Geometry: final body of the model. Coordinates: model frame, mm. A direction names the side the tool comes from. Coordinates: 2 decimals unless noted, no trailing zeros. Order: outer loops, then holes, each group sorted by start corner. A loop starts at its lowest first (then second) coordinate and runs counter-clockwise, first axis right, second up. Notation, with made-up numbers: (18, -5) - (34, -5) arc R31 cw to (34, 25) - close; hole circle Ø1 at (-28.75, 28.25). An arc over 180 degrees is marked (long way). Use a Markdown table: item, result. Add a question column.
```python
from build123d import *

# Parameters (mm, degrees)
F0_W     = 49
F0_H     = 49
F0_W_2   = 41
F0_H_2   = 41
F1_DEPTH = 20
F2_DEPTH = 10
F3_D     = 5.5
F5_D     = 5.5
F7_DEPTH = 5


with BuildPart() as f1:
    # F0 (on Front) → F1 (new body)
    with BuildSketch(Plane.XZ):
        Rectangle(F0_W, F0_H)
        Rectangle(F0_W_2, F0_H_2, mode=Mode.SUBTRACT)
    extrude(amount=F1_DEPTH)

    # F0 (on Front) → F2 (join)
    with BuildSketch(Plane.XZ):
        Rectangle(F0_W, F0_H)
        Rectangle(F0_W_2, F0_H_2, mode=Mode.SUBTRACT)
        Rectangle(F0_W_2, F0_H_2)
    extrude(amount=-F2_DEPTH)

    # F3 (through all)
    with Locations(Plane.XZ):
        with Locations((0, 10), (0, -10)):
            Hole(F3_D / 2)

    # F5 (through all)
    with Locations(Plane.YZ.offset(24.5)):
        with Locations((-10, 0)):
            Hole(F5_D / 2)


with BuildPart() as f7:
    # F6 (on face) → F7 (new body)
    with BuildSketch(Plane.XZ):
        Polygon((5.1, 10), (2.55, 14.4167295593), (-2.55, 14.4167295593), (-5.1, 10), (-2.55, 5.5832704407), (2.55, 5.5832704407), align=None)
    extrude(amount=-F7_DEPTH)


with BuildPart() as f7b:
    # F6 (on face) → F7, piece 2 (new body)
    with BuildSketch(Plane.XZ):
        Polygon((5.1, -10), (2.55, -5.5832704407), (-2.55, -5.5832704407), (-5.1, -10), (-2.55, -14.4167295593), (2.55, -14.4167295593), align=None)
    extrude(amount=-F7_DEPTH)


with BuildPart() as f1_1:
    add(f1.part)

    # F8: cut F7, F7b
    add(f7.part, mode=Mode.SUBTRACT)
    add(f7b.part, mode=Mode.SUBTRACT)


solid = f1_1.part
```
1) Line query: line 1 (Z direction, x = 0, y = 8.05); line 2 (Z direction, x = -15, y = -10.5). Output: solid intervals per line, ascending. Write a range as from..to.
2) Access query for faces 4 (the flat face through (0, -10, 20.5)), 5 (the flat face through (21, -20, 0)). Directions: +Z, -Z, +X, -X, +Y, -Y. A direction counts if a zero-diameter tool reaches every point of the face in a straight line with its end or side. Return the directions, or none.
3) Section query A-A (x = 0). Return the cut outline in (y, z).
4) Section query B-B (y = -10). Return the cut outline in (x, z).
5) Section query D-D (x = -14). Return the cut outline in (y, z).
6) First-contact query: pin 1 (7 mm diameter, centred on x = 0, z = 10, fed in from -Y); pin 2 (8 mm diameter, centred on x = -13, z = -16, fed in from -Y); pin 3 (2.5 mm diameter, centred on x = 1, z = 10.5, fed in from -Y). Flat tips, straight axial feed; report the tip coordinate or a pass-through.
7) Section query C-C (z = 0). Return the cut outline in (x, y), and give its area (3 significant figures).
8) Draft query along Y for faces 1 (the flat face through (-20.5, -5, 0)), 2 (the flat face through (2.2, 5, 8.1)), 3 (the cylindrical face through (-22.53, -12.54, -1.05)). Return one class per face: released by +Y, released by -Y, zero draft, split by the parting line, or undercut.
From the geometry:
| question | item | result |
|---|---|---|
| 1 | line 1 | z = -24.5..-12.75, -7.25..7.25, 12.75..24.5 |
| 1 | line 2 | z = -24.5..-20.5, 20.5..24.5 |
| 2 | face 4 | -Y |
| 2 | face 5 | +Z, -Z, +X, -X, -Y |
| 3 | outline | (-20, -24.5) - (10, -24.5) - (10, -12.75) - (5, -12.75) - (5, -14.42) - (0, -14.42) - (0, -20.5) - (-20, -20.5) - close; (-20, 20.5) - (0, 20.5) - (0, 14.42) - (5, 14.42) - (5, 12.75) - (10, 12.75) - (10, 24.5) - (-20, 24.5) - close; (0, -5.58) - (5, -5.58) - (5, -7.25) - (10, -7.25) - (10, 7.25) - (5, 7.25) - (5, 5.58) - (0, 5.58) - close |
| 4 | outline | (-24.5, -24.5) - (24.5, -24.5) - (24.5, -2.75) - (20.5, -2.75) - (20.5, -20.5) - (-20.5, -20.5) - (-20.5, -2.75) - (-24.5, -2.75) - close; (-24.5, 2.75) - (-20.5, 2.75) - (-20.5, 20.5) - (20.5, 20.5) - (20.5, 2.75) - (24.5, 2.75) - (24.5, 24.5) - (-24.5, 24.5) - close |
| 5 | outline | (-20, -24.5) - (10, -24.5) - (10, 24.5) - (-20, 24.5) - (-20, 20.5) - (0, 20.5) - (0, -20.5) - (-20, -20.5) - close |
| 6 | pin 1 | stops at y = 5 |
| 6 | pin 2 | stops at y = 0 |
| 6 | pin 3 | passes through |
| 7 | outline | (-24.5, -20) - (-20.5, -20) - (-20.5, -12.75) - (-24.5, -12.75) - close; (-24.5, -7.25) - (-20.5, -7.25) - (-20.5, 0) - (20.5, 0) - (20.5, -7.25) - (24.5, -7.25) - (24.5, 10) - (-24.5, 10) - close; (20.5, -20) - (24.5, -20) - (24.5, -12.75) - (20.5, -12.75) - close |
| 7 | area | 606 mm^2 |
| 8 | face 1 | zero draft |
| 8 | face 2 | released by -Y |
| 8 | face 3 | undercut |
